The model under review builds one solid part; all positions refer to its coordinate system, in mm. Face numbers are marked on the shaded views. Round coordinates to 2 decimals unless told otherwise and drop trailing zeros. Order: outer loops, then holes, each group sorted by start corner. A loop starts at its lowest first (then second) coordinate and runs counter-clockwise, first axis right, second up. Notation, with made-up numbers: M 56,-23 L 64,-23 A14 cw 64,-18 Z; hole C 69.25,-14 d11. An arc over 180 degrees is marked long. Answer as CSV lines item,"result". Start each with the question number.
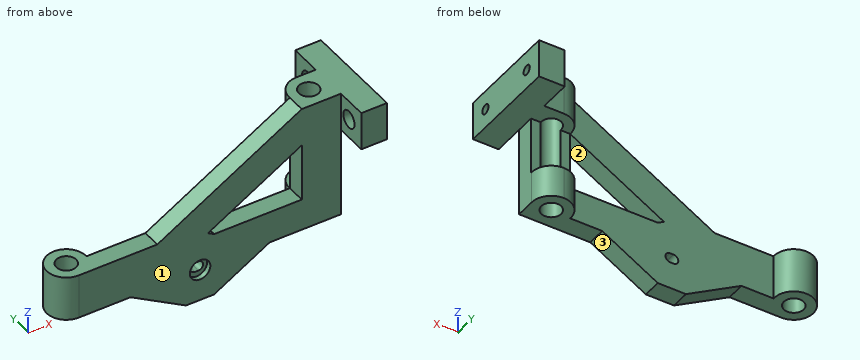
from build123d import *
from build123d.topology import SkipClean

# Parameters (mm, degrees)
SKETCH_2_R           = 3.05
SKETCH_2_R_2         = 1.55
EXTRUDE_1_DEPTH      = 25
CUT_EXTRUDE_3_DEPTH  = 74.430746455
SKETCH_8_R           = 1.6
CUT_EXTRUDE_4_DEPTH  = 0.8
CUT_EXTRUDE_START    = -2.895
CUT_EXTRUDE_10_DEPTH = 6.1
SKETCH_21_W          = 6
SKETCH_21_H          = 16
EXTRUDE_9_DEPTH      = 4
SKETCH_22_R          = 0.75
CUT_EXTRUDE_16_DEPTH = 4
CUT_EXTRUDE_19_DEPTH = 76.099311082
CUT_EXTRUDE_21_REACH = 87.974
SKETCH_25_W          = 9
SKETCH_25_H          = 3.205
CUT_EXTRUDE_22_REACH = 42.469
SKETCH_27_R          = 1.35
CUT_EXTRUDE_23_DEPTH = 2


# Read off the part's stored shape, not the designer's step: 切除-拉伸10
with BuildPart() as part:
    # 草图2 → 凸台-拉伸1 (new body)
    # profile 1 of 8: a face of its own
    with SkipClean():  # the faces are left unmerged after this step: merging them gives an invalid solid
        with BuildSketch(Plane.XY.offset(70)):
            with Locations((-18.9, 15.755)):
                Circle(SKETCH_2_R)
            with Locations((-18.9, 15.755)):
                Circle(SKETCH_2_R_2, mode=Mode.SUBTRACT)
        # profile 2 of 8: a face of its own
        with BuildSketch(Plane.XY.offset(70)):
            with BuildLine():
                Line((0, 12.705), (0, 15.6))
                Line((0, 15.6), (-15.853941071, 15.6))
                ThreePointArc((-15.853941071, 15.6), (-16.798839606, 13.544202633), (-18.9, 12.705))
                Line((-18.9, 12.705), (0, 12.705))
            make_face()
        # profile 3 of 8: a face of its own
        with BuildSketch(Plane.XY.offset(70)):
            with BuildLine():
                Line((15.853941071, 15.6), (0, 15.6))
                Line((0, 15.6), (0, 12.705))
                Line((0, 12.705), (18.9, 12.705))
                ThreePointArc((18.9, 12.705), (16.798839606, 13.544202633), (15.853941071, 15.6))
            make_face()
        # profile 4 of 8: a face of its own
        with BuildSketch(Plane.XY.offset(70)):
            with Locations((18.9, 15.755)):
                Circle(SKETCH_2_R)
            with Locations((18.9, 15.755)):
                Circle(SKETCH_2_R_2, mode=Mode.SUBTRACT)
        # profile 5 of 8: a face of its own
        with BuildSketch(Plane.XY.offset(70)):
            with BuildLine():
                Line((21.95, 18.805), (18.9, 18.805))
                ThreePointArc((18.9, 18.805), (21.056675683, 17.911675683), (21.95, 15.755))
                Line((21.95, 15.755), (21.95, 18.805))
            make_face()
        # profile 6 of 8: a face of its own
        with BuildSketch(Plane.XY.offset(70)):
            with BuildLine():
                ThreePointArc((18.9, 18.805), (16.689202633, 17.856160394), (15.853941071, 15.6))
                ThreePointArc((15.853941071, 15.6), (16.798839606, 13.544202633), (18.9, 12.705))
                Line((18.9, 12.705), (18.9, 14.205))
                ThreePointArc((18.9, 14.205), (17.35, 15.755), (18.9, 17.305))
                Line((18.9, 17.305), (18.9, 18.805))
            make_face()
        # profile 7 of 8: a face of its own
        with BuildSketch(Plane.XY.offset(70)):
            with BuildLine():
                Line((18.9, 14.205), (18.9, 12.705))
                ThreePointArc((18.9, 12.705), (21.056675683, 13.598324317), (21.95, 15.755))
                ThreePointArc((21.95, 15.755), (21.056675683, 17.911675683), (18.9, 18.805))
                Line((18.9, 18.805), (18.9, 17.305))
                ThreePointArc((18.9, 17.305), (19.996015511, 16.851015511), (20.45, 15.755))
                ThreePointArc((20.45, 15.755), (19.996015511, 14.658984489), (18.9, 14.205))
            make_face()
        # profile 8 of 8: a face of its own
        with BuildSketch(Plane.XY.offset(70)):
            with BuildLine():
                ThreePointArc((21.95, 15.755), (21.056675683, 13.598324317), (18.9, 12.705))
                Line((18.9, 12.705), (21.95, 12.705))
                Line((21.95, 12.705), (21.95, 15.755))
            make_face()
        extrude(amount=-EXTRUDE_1_DEPTH)

    # 草图7 → 切除-拉伸3 (cut, through all)
    with SkipClean():  # the faces are left unmerged after this step: merging them gives an invalid solid
        with BuildSketch(Plane(origin=(0, 15.6, 0), x_dir=(1, 0, 0), z_dir=(0, 1, 0))):
            with BuildLine():
                Line((0.25, -50.75), (-0.25, -50.75))
                ThreePointArc((-0.25, -50.75), (-1, -50), (-0.25, -49.25))
                Line((-0.25, -49.25), (0.25, -49.25))
                ThreePointArc((0.25, -49.25), (1, -50), (0.25, -50.75))
            make_face()
        extrude(amount=-CUT_EXTRUDE_3_DEPTH, mode=Mode.SUBTRACT)

    # 草图8 → 切除-拉伸4 (cut)
    with SkipClean():  # the faces are left unmerged after this step: merging them gives an invalid solid
        with BuildSketch(Plane.XZ.offset(-12.705)):
            with Locations((0, 50)):
                Circle(SKETCH_8_R)
        extrude(amount=-CUT_EXTRUDE_4_DEPTH, mode=Mode.SUBTRACT)

    # 切除-拉伸10 outline → 切除-拉伸10 (cut)
    with SkipClean():  # the faces are left unmerged after this step: merging them gives an invalid solid
        with BuildSketch(Plane(origin=(0, 15.6, 0), x_dir=(1, 0, 0), z_dir=(0, 1, 0)).offset(CUT_EXTRUDE_START)):
            Polygon((-6.666660498, -57), (-21.95, -57), (-21.95, -70), (15.85, -70), align=None)
            Polygon((-21.95, -50), (-10.853941071, -50), (-2.193687033, -45), (-21.95, -45), align=None)
            Polygon((10.853941071, -50), (21.95, -50), (21.95, -45), (2.193687033, -45), align=None)
        extrude(amount=CUT_EXTRUDE_10_DEPTH, mode=Mode.SUBTRACT)

    # 草图21 → 凸台-拉伸9 (add)
    with SkipClean():  # the faces are left unmerged after this step: merging them gives an invalid solid
        with BuildSketch(Plane(origin=(21.95, 0, 0), x_dir=(0, 0, -1), z_dir=(1, 0, 0))):
            with Locations((-67, 15.755)):
                Rectangle(SKETCH_21_W, SKETCH_21_H)
        extrude(amount=EXTRUDE_9_DEPTH)

    # 草图22 → 切除-拉伸16 (cut)
    with SkipClean():  # the faces are left unmerged after this step: merging them gives an invalid solid
        with BuildSketch(Plane(origin=(25.95, 0, 0), x_dir=(0, 0, -1), z_dir=(1, 0, 0))):
            with Locations((-67, 20.755)):
                Circle(SKETCH_22_R)
            with Locations((-67, 10.755)):
                Circle(SKETCH_22_R)
        extrude(amount=-CUT_EXTRUDE_16_DEPTH, mode=Mode.SUBTRACT)

    # 草图23 → 切除-拉伸19 (cut, through all)
    with SkipClean():  # the faces are left unmerged after this step: merging them gives an invalid solid
        with BuildSketch(Plane(origin=(0, 15.6, 0), x_dir=(1, 0, 0), z_dir=(0, 1, 0))):
            Polygon((1.227614882, -55.557762016), (15.85, -64), (15.85, -55), (2.193687033, -55), align=None)
        extrude(amount=-CUT_EXTRUDE_19_DEPTH, mode=Mode.SUBTRACT)

    # 草图25 → 切除-拉伸21 (cut, up to next)
    with BuildSketch(Plane(origin=(21.95, 0, 0), x_dir=(0, 0, -1), z_dir=(1, 0, 0)), mode=Mode.PRIVATE) as cut_extrude_21_sk1:
        with Locations((-59.5, 17.2025)):
            Rectangle(SKETCH_25_W, SKETCH_25_H)
    cut_extrude_21_tool1 = extrude(cut_extrude_21_sk1.sketch, amount=-CUT_EXTRUDE_21_REACH, mode=Mode.PRIVATE) & part.part
    add(cut_extrude_21_tool1.solids().sort_by_distance((21.95, 17.2025, 59.5))[0], mode=Mode.SUBTRACT)

    # 草图26 → 切除-拉伸22 (cut, up to next)
    with BuildSketch(Plane(origin=(0, 0, 50), x_dir=(-1, 0, 0), z_dir=(0, 0, -1)), mode=Mode.PRIVATE) as cut_extrude_22_sk1:
        with BuildLine():
            ThreePointArc((-21.95, 15.755), (-21.056675683, 17.911675683), (-18.9, 18.805))
            Line((-18.9, 18.805), (-21.95, 18.805))
            Line((-21.95, 18.805), (-21.95, 15.755))
        make_face()
    cut_extrude_22_tool1 = extrude(cut_extrude_22_sk1.sketch, amount=-CUT_EXTRUDE_22_REACH, mode=Mode.PRIVATE) & part.part
    add(cut_extrude_22_tool1.solids().sort_by_distance((21.268728, 18.123728, 50))[0], mode=Mode.SUBTRACT)

    # 草图27 → 切除-拉伸23 (cut)
    with SkipClean():  # the faces are left unmerged after this step: merging them gives an invalid solid
        with BuildSketch(Plane.ZY.offset(-21.95)):
            with Locations((67, 20.755)):
                Circle(SKETCH_27_R)
            with Locations((67, 10.755)):
                Circle(SKETCH_27_R)
        extrude(amount=-CUT_EXTRUDE_23_DEPTH, mode=Mode.SUBTRACT)


solid = part.part
Item 1: Wall thickness on probe 1 along Y at (x, z) = (24.7, 67) (3 decimals); probe 2 along Y at (x, z) = (22.65, 67) (3 decimals); probe 3 along Y at (x, z) = (-18.9, 55) (3 decimals): over which ranges is each line inside the solid? List them lowest first. Write a range as [from, to].
Item 2: The part is to be moulded in two halves that separate along Z. For the marked faces 1, 2 and 3, say which applies: +Z half, -Z half, draft (parallel to the pull), parting line (faces both ways), or undercut.
Item 3: For pin 1 (3 mm diameter, centred on x = 17, y = 17, fed in from -Z); pin 2 (3 mm diameter, centred on x = -16, z = 59, fed in from -Y); pin 3 (1 mm diameter, centred on y = 14.5, z = 52, fed in from +X); pin 4 (2 mm diameter, centred on y = 20.755, z = 67, fed in from -X), all flat-tipped, find the tip position at first contact; note any pin that passes through.
Item 4: Consider section A-A (z = 63). State the section outline as (x, y) points (3 decimals).
Item 5: Consider section B-B (x = 12.5). State the section outline as (y, z) points (3 decimals).
Item 6: Consider section C-C (x = -4.5). State the section outline as (y, z) points (3 decimals), and give its area (3 significant figures).
Reported:
1,probe 1,"y = [7.755, 10.005], [11.505, 20.005], [21.505, 23.755]"
1,probe 2,"y = [7.755, 9.405], [12.105, 19.405], [22.105, 23.755]"
1,probe 3,"y = [12.705, 14.205], [17.305, 18.805]"
2,face 1,"draft"
2,face 2,"undercut"
2,face 3,"-Z half"
3,pin 1,"stops at z = 50"
3,pin 2,"passes through"
3,pin 3,"stops at x = 21.95"
3,pin 4,"stops at x = 23.95"
4,outline,"M 3.726,12.705 L 14.118,12.705 L 14.118,15.6 L 3.726,15.6 Z; M 15.85,12.705 L 21.95,12.705 L 21.95,15.6 L 20.442,15.6 A1.55 cw 17.358,15.6 L 15.85,15.6 Z"
5,outline,"M 12.705,50 L 15.6,50 L 15.6,55 L 12.705,55 Z; M 12.705,62.066 L 15.6,62.066 L 15.6,68.066 L 12.705,68.066 Z"
6,outline,"M 12.705,46.332 L 15.6,46.332 L 15.6,58.251 L 12.705,58.251 Z"
6,area,"34.5 mm²"
